```python
from build123d import *

# Parameters (mm, degrees)
EXTRUDE_1_DEPTH     = 8
CUT_EXTRUDE_1_DEPTH = 1
FILLET_1_R          = 1
HOLE_WIZARD_M3_1_D  = 3.2


with BuildPart() as part:
    # ｽｹｯﾁ1 → ﾎﾞｽ - 押し出し1 (new body)
    with BuildSketch(Plane.XY):
        with BuildLine():
            Line((-128.683849372, 3.5), (128.683849372, 3.5))
            ThreePointArc((128.683849372, 3.5), (131.158723106, 2.474873734), (132.183849372, 0))
            Line((132.183849372, 0), (132.183849372, -20))
            ThreePointArc((132.183849372, -20), (128.945217461, -23.490227317), (125.222885531, -20.521276596))
            ThreePointArc((125.222885531, -20.521276596), (118.492510756, -8.341265421), (105.445949295, -3.5))
            Line((105.445949295, -3.5), (-105.445949295, -3.5))
            ThreePointArc((-105.445949295, -3.5), (-118.492510756, -8.341265421), (-125.222885531, -20.521276596))
            ThreePointArc((-125.222885531, -20.521276596), (-128.945217461, -23.490227317), (-132.183849372, -20))
            Line((-132.183849372, -20), (-132.183849372, 0))
            ThreePointArc((-132.183849372, 0), (-131.158723106, 2.474873734), (-128.683849372, 3.5))
        make_face()
    extrude(amount=-EXTRUDE_1_DEPTH)

    # ｽｹｯﾁ1<4> → ｶｯﾄ - 押し出し1 (cut)
    with BuildSketch(Plane.XY):
        with BuildLine():
            ThreePointArc((-125.183849372, 0), (-126.208975638, 2.474873734), (-128.683849372, 3.5))
            ThreePointArc((-128.683849372, 3.5), (-131.158723106, 2.474873734), (-132.183849372, 0))
            Line((-132.183849372, 0), (-132.183849372, -20))
            ThreePointArc((-132.183849372, -20), (-128.945217461, -23.490227317), (-125.222885531, -20.521276596))
            ThreePointArc((-125.222885531, -20.521276596), (-125.203758298, -20.396939676), (-125.183849372, -20.272725524))
            Line((-125.183849372, -20.272725524), (-125.183849372, 0))
        make_face()
        with BuildLine():
            Line((125.183849372, 0), (125.183849372, -20.272725524))
            ThreePointArc((125.183849372, -20.272725524), (125.203758298, -20.396939676), (125.222885531, -20.521276596))
            ThreePointArc((125.222885531, -20.521276596), (128.945217461, -23.490227317), (132.183849372, -20))
            Line((132.183849372, -20), (132.183849372, 0))
            ThreePointArc((132.183849372, 0), (131.158723106, 2.474873734), (128.683849372, 3.5))
            ThreePointArc((128.683849372, 3.5), (126.208975638, 2.474873734), (125.183849372, 0))
        make_face()
    extrude(amount=-CUT_EXTRUDE_1_DEPTH, mode=Mode.SUBTRACT)

    # ﾌｨﾚｯﾄ1
    fillet_1_edges = [part.edges().sort_by_distance(p)[0] for p in [
        (-128.683849372, 3.5, -0.5),
        (-125.183849372, -20.272725524, -0.5),
        (128.683849372, 3.5, -0.5),
        (125.183849372, -20.272725524, -0.5),
    ]]
    fillet(fillet_1_edges, radius=FILLET_1_R - 0.0001)  # a hair under: the kernel refuses the full size

    # M3 すきま穴1 (through all)
    with Locations(Plane(origin=(-128.683849372, -20, -8), x_dir=(-1, 0, 0), z_dir=(0, 0, -1))):
        with Locations((0, 0), (0, 20), (-48.683849372, 20), (-257.367698744, 0), (-257.367698744, 20), (-208.683849372, 20)):
            Hole(HOLE_WIZARD_M3_1_D / 2)


solid = part.part
```
Check sheet for the modelled part. Datum: model origin and axes. Units: mm. A direction names the side the tool comes from. Round coordinates to 2 decimals unless told otherwise and drop trailing zeros. Order: outer loops, then holes, each group sorted by start corner. A loop starts at its lowest first (then second) coordinate and runs counter-clockwise, first axis right, second up. Notation, with made-up numbers: (54, 27.5) -> (88, 27.5) arc R4 ccw to (88, 32.5) -> close; hole circle Ø6 at (4, 58). An arc over 180 degrees is marked (long way). One line per item, written item: value. Start each with the question number.
Q1. Cross-section at A-A (z = -4.5). Record the boundary of the cut face in (x, y), and give its area (3 significant figures).
Q2. Cross-section at C-C (x = 32). Record the boundary of the cut face in (y, z).
Q3. Thickness scan on line 1 (Y direction, x = -80, z = -4.5); line 2 (X direction, y = -21.25, z = -1.75); line 3 (Y direction, x = -22.5, z = -5.5). Record the ranges inside material, lowest first.
Q4. Gauge pin test, flat ends, axial feed: pin 1 Ø1.5 at (x, z) = (40, -5) entering from -Y; pin 2 Ø0.5 at (y, z) = (-8, -0.5) entering from -X; pin 3 Ø4 at (x, y) = (128.68, -20) entering from +Z. Record the tip position at first contact, or that the pin passes through.
Q5. Set-up check for faces 5 (the face through (118.64, -8.47, -3.94)), 6 (the face through (1, -3, -8)): record each of +Z, -Z, +X, -X, +Y, -Y from which the full face is reachable in a straight line by a thin tool's end or side.
Q6. Mould release check, pull along X, two halves, no side actions. Record for faces 1 (the face through (-118.34, -8.21, -3.94)), 2 (the face through (-132.184, -10, -4)), 3 (the face through (132.184, -10, -4)), 4 (the face through (129.018, -23.484, -4.451)): pulls with the +X half, pulls with the -X half, needs draft (parallel to the pull), parting line crosses it, or undercut.
Q7. Cross-section at D-D (x = -115.5). Record the boundary of the cut face in (y, z).
Q8. Cross-section at B-B (y = -11.75). Record the boundary of the cut face in (x, z), and give its area (3 significant figures).
Completed:
1. outline: (-132.18, -20) arc R3.5 ccw to (-125.22, -20.52) arc R20 cw to (-105.45, -3.5) -> (105.45, -3.5) arc R20 cw to (125.22, -20.52) arc R3.5 ccw to (132.18, -20) -> (132.18, 0) arc R3.5 ccw to (128.68, 3.5) -> (-128.68, 3.5) arc R3.5 ccw to (-132.18, 0) -> close; hole circle Ø3.2 at (-128.68, -20); hole circle Ø3.2 at (-128.68, 0); hole circle Ø3.2 at (-80, 0); hole circle Ø3.2 at (80, 0); hole circle Ø3.2 at (128.68, -20); hole circle Ø3.2 at (128.68, 0)
1. area: 2,230 mm²
2. outline: (-3.5, -8) -> (3.5, -8) -> (3.5, 0) -> (-3.5, 0) -> close
3. line 1: y = -3.5 to -1.6, 1.6 to 3.5
3. line 2: x = -131.95 to -129.68, -127.69 to -125.41, 125.41 to 127.69, 129.68 to 131.95
3. line 3: y = -3.5 to 3.5
4. pin 1: stops at y = -3.5
4. pin 2: stops at x = -125.18
4. pin 3: stops at z = -1
5. face 5: +Z, -Z, -Y
5. face 6: -Z, +X, -X, +Y, -Y
6. face 1: undercut
6. face 2: pulls with the -X half
6. face 3: pulls with the +X half
6. face 4: undercut
7. outline: (-6.21, -8) -> (3.5, -8) -> (3.5, 0) -> (-6.21, 0) -> close
8. outline: (-132.18, -8) -> (-121.63, -8) -> (-121.63, 0) -> (-125.18, 0) -> (-125.18, -1) -> (-132.18, -1) -> close; (121.63, -8) -> (132.18, -8) -> (132.18, -1) -> (125.18, -1) -> (125.18, 0) -> (121.63, 0) -> close
8. area: 155 mm²
